from build123d import *

# Parameters (mm, degrees)
SKETCH_W        = 150
SKETCH_H        = 100
PAD_DEPTH       = 4
SKETCH005_W     = 5
SKETCH005_H     = 100
PAD001_DEPTH    = 18
SKETCH007_R     = 3.5
POCKET001_DEPTH = 5
SKETCH006_R     = 2.875
PAD002_DEPTH    = 7
SKETCH008_W     = 16
SKETCH008_H     = 18
POCKET_DEPTH    = 5
SKETCH009_W     = 16
SKETCH009_H     = 18
POCKET002_DEPTH = 5


with BuildPart() as part:
    # Sketch → Pad (new body)
    with BuildSketch(Plane.XY):
        Rectangle(SKETCH_W, SKETCH_H)
    extrude(amount=PAD_DEPTH)

    # Sketch005 → Pad001 (join)
    with BuildSketch(Plane.XY.offset(4)):
        with Locations((-72.5, 0)):
            Rectangle(SKETCH005_W, SKETCH005_H)
        with Locations((72.5, 0)):
            Rectangle(SKETCH005_W, SKETCH005_H)
    extrude(amount=PAD001_DEPTH)

    # Sketch007 → Pocket001 (cut)
    with BuildSketch(Plane.XY.offset(4)):
        with Locations((-26, 42.5)):
            Circle(SKETCH007_R)
        with Locations((27.5, 42.5)):
            Circle(SKETCH007_R)
        with Locations((27.5, -42.5)):
            Circle(SKETCH007_R)
        with Locations((-26, -42.5)):
            Circle(SKETCH007_R)
    extrude(amount=-POCKET001_DEPTH, mode=Mode.SUBTRACT)

    # Sketch006 (on Face6 of Pad001) → Pad002 (join)
    with BuildSketch(Plane.XY.offset(4)):
        with Locations((-59, 44.1)):
            Circle(SKETCH006_R)
        with Locations((-5.5, 44.1)):
            Circle(SKETCH006_R)
        with Locations((48, 44.1)):
            Circle(SKETCH006_R)
        with Locations((48.2, -44.1)):
            Circle(SKETCH006_R)
        with Locations((-5.3, -44.1)):
            Circle(SKETCH006_R)
        with Locations((-58.8, -44.1)):
            Circle(SKETCH006_R)
    extrude(amount=PAD002_DEPTH)

    # Sketch008 (on Face9 of Pad002) → Pocket (cut)
    with BuildSketch(Plane(origin=(-75, 0, 0), x_dir=(0, -1, 0), z_dir=(-1, 0, 0))):
        with Locations((-42, 13)):
            Rectangle(SKETCH008_W, SKETCH008_H)
        with Locations((42, 13)):
            Rectangle(SKETCH008_W, SKETCH008_H)
    extrude(amount=-POCKET_DEPTH, mode=Mode.SUBTRACT)

    # Sketch009 (on Face11 of Pocket) → Pocket002 (cut)
    with BuildSketch(Plane.YZ.offset(75)):
        with Locations((42, 13)):
            Rectangle(SKETCH009_W, SKETCH009_H)
        with Locations((-42, 13)):
            Rectangle(SKETCH009_W, SKETCH009_H)
    extrude(amount=-POCKET002_DEPTH, mode=Mode.SUBTRACT)


solid = part.part
Build history of the part. All positions in model axes, mm. A direction names the side the tool comes from. Coordinates: 2 decimals unless noted, no trailing zeros. Write each loop counter-clockwise with the first axis right and the second up, starting at its lowest first coordinate (ties: lowest second). Pieces come first, ordered by that corner, then holes.
(1) Cut at A-A on x = -26. List the corners of the cut face in (y, z), and give its area (3 significant figures).
(2) Pin check, flat tips, straight feed: pin 1 Ø3 at (x, y) = (-4.5, 45.5) entering from +Z; pin 2 Ø2.5 at (x, z) = (72, 8.5) entering from -Y; pin 3 Ø1 at (x, y) = (-14, -32) entering from +Z. Stop position of each tip, or through.
(3) Mould opens along X. For faces 4 (the flat face through (-59, 44, 11)), 5 (the flat face through (75, -1, 11)), 6 (the flat face through (70, 0, 13)) say: pulls with the +X half, pulls with the -X half, needs draft (parallel to the pull), parting line crosses it, or undercut.
(4) Cut at C-C on y = 44.1. List the corners of the cut face in (x, z) (3 decimals).
(5) Drill centre lines: line 1 (Y direction, x = 27.5, z = 1.85); line 2 (X direction, y = 5.5, z = 6.75); line 3 (Z direction, x = -55, y = -34.5). Where is each one in solid material? Low to high.
(6) Cut at B-B on z = 5.5. List the corners of the cut face in (x, y) (3 decimals).
(7) 3-axis set-ups, long thin cutter, end or side, ignore diameter. For faces 1 (the flat face through (48, -44, 11)), 2 (the flat face through (73, 34, 13)), 3 (the cylindrical face through (-3.97, -46.65, 7.45)): which of +Z, -Z, +X, -X, +Y, -Y reach the whole face in a straight line?
(8) Cut at D-D on y = -13. List the corners of the cut face in (x, z), and give its area (3 significant figures).
Working result:
1. outline: (-50, 0) - (-46, 0) - (-46, 4) - (-50, 4) - close; (-39, 0) - (39, 0) - (39, 4) - (-39, 4) - close; (46, 0) - (50, 0) - (50, 4) - (46, 4) - close
1. area: 344 mm2
2. pin 1: stops at z = 11
2. pin 2: stops at y = -34
2. pin 3: stops at z = 4
3. face 4: needs draft
3. face 5: pulls with the +X half
3. face 6: undercut
4. outline: (-75, 0) - (-29.113, 0) - (-29.113, 4) - (-56.125, 4) - (-56.125, 11) - (-61.875, 11) - (-61.875, 4) - (-75, 4) - close; (-22.887, 0) - (24.387, 0) - (24.387, 4) - (-2.625, 4) - (-2.625, 11) - (-8.375, 11) - (-8.375, 4) - (-22.887, 4) - close; (30.613, 0) - (75, 0) - (75, 4) - (50.875, 4) - (50.875, 11) - (45.125, 11) - (45.125, 4) - (30.613, 4) - close
5. line 1: y = -50 to -46, -39 to 39, 46 to 50
5. line 2: x = -75 to -70, 70 to 75
5. line 3: z = 0 to 4
6. outline: (-75, -34) - (-70, -34) - (-70, 34) - (-75, 34) - close; circle Ø5.75 at (-59, 44.1); circle Ø5.75 at (-58.8, -44.1); circle Ø5.75 at (-5.5, 44.1); circle Ø5.75 at (-5.3, -44.1); circle Ø5.75 at (48, 44.1); circle Ø5.75 at (48.2, -44.1); (70, -34) - (75, -34) - (75, 34) - (70, 34) - close
7. face 1: +Z, +X, -X, +Y, -Y
7. face 2: +Z, +X, -X, +Y
7. face 3: +Z
8. outline: (-75, 0) - (75, 0) - (75, 22) - (70, 22) - (70, 4) - (-70, 4) - (-70, 22) - (-75, 22) - close
8. area: 780 mm2
